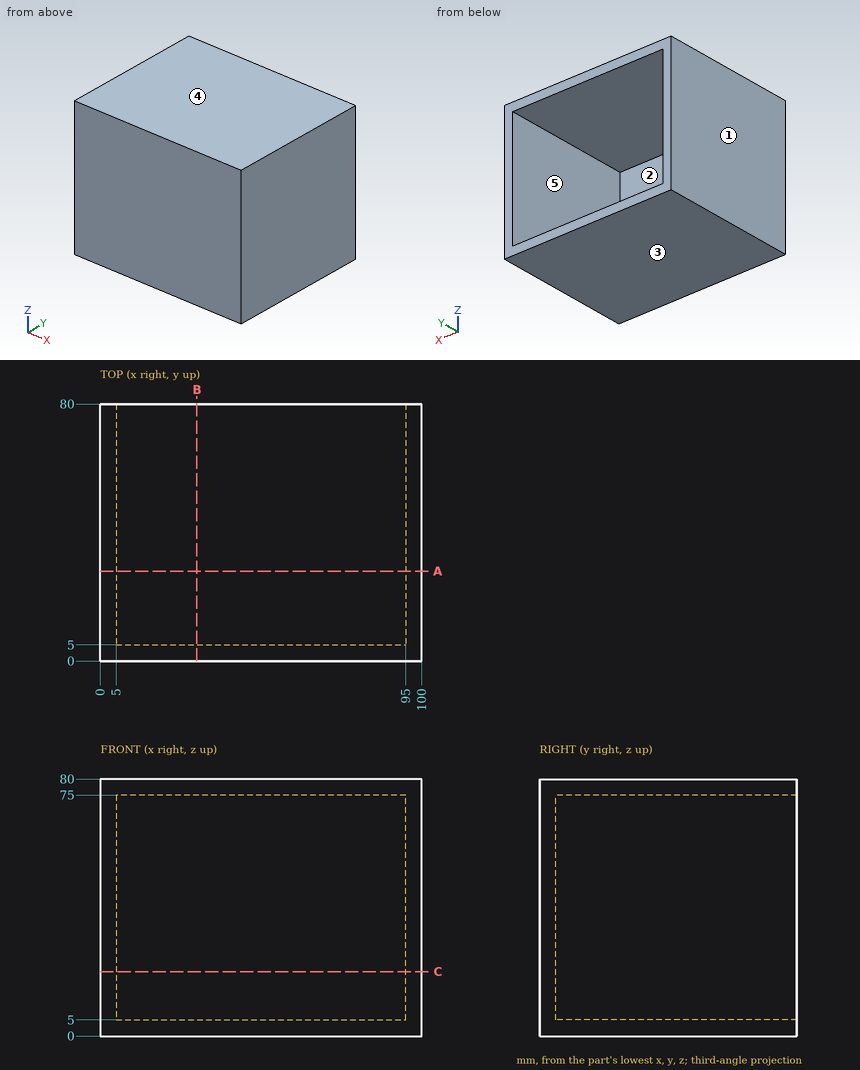
Geometry check sheet. Reference: drawing and pictorial views, mm from the part's lowest x, y, z. A direction names the side the tool comes from. Give positions to 0.01 mm unless a question says otherwise; leave off trailing zeros. Order: outer loops, then holes, each group sorted by start corner. A loop starts at its lowest first (then second) coordinate and runs counter-clockwise, first axis right, second up. Notation, with made-up numbers: M -29.5,10.25 L -8.5,10.25 A20 ccw -8.5,36.25 Z; hole C 30.25,28.5 d2. An arc over 180 degrees is marked long. Answer in a Markdown table with one row per item.
1) Cross-section at A-A, the plane y = 28. Enter the section's corners in (x, z).
Filled sheet:
| item | result |
|---|---|
| outline | M 0,0 L 100,0 L 100,80 L 0,80 Z; hole M 5,5 L 95,5 L 95,75 L 5,75 Z |
2) Thickness scan on L1, parallel to Z at x = 54.5, y = 44.5; L2, parallel to X at y = 75, z = 19; L3, parallel to Y at x = 91.5, z = 59. Record the ranges inside material, lowest first. Write a range as [from, to].
Filled sheet:
| item | result |
|---|---|
| L1 | z = [0, 5], [75, 80] |
| L2 | x = [0, 5], [95, 100] |
| L3 | y = [0, 5] |
3) Cross-section at C-C, the plane z = 20. Enter the section's corners in (x, y), plus the area to 3 significant figures.
Filled sheet:
| item | result |
|---|---|
| outline | M 0,0 L 100,0 L 100,80 L 95,80 L 95,5 L 5,5 L 5,80 L 0,80 Z |
| area | 1,250 mm2 |
4) Access from +Z, -Z, +X, -X, +Y, -Y to the whole of each face (thin tool, end or side, straight path). Record for the marked faces 4 and 5.
Filled sheet:
| item | result |
|---|---|
| face 4 | +Z, +X, -X, +Y, -Y |
| face 5 | +Y |
5) Gauge pin test, flat end, axial feed: P1, Ø21, axis at x = 30, z = 46, coming from the +Y side. Record the tip position at first contact, or that the pin passes through.
Filled sheet:
| item | result |
|---|---|
| P1 | stops at y = 5 |
6) Cross-section at B-B, the plane x = 30. Enter the section's corners in (y, z), plus the area to 3 significant figures.
Filled sheet:
| item | result |
|---|---|
| outline | M 0,0 L 80,0 L 80,5 L 5,5 L 5,75 L 80,75 L 80,80 L 0,80 Z |
| area | 1,150 mm2 |
7) Release check for a two-part mould opening along Z. For the marked faces 1, 2 and 3 record: +Z half, -Z half, draft (parallel to the pull), parting line (faces both ways), or undercut.
Filled sheet:
| item | result |
|---|---|
| face 1 | draft |
| face 2 | undercut |
| face 3 | -Z half |
